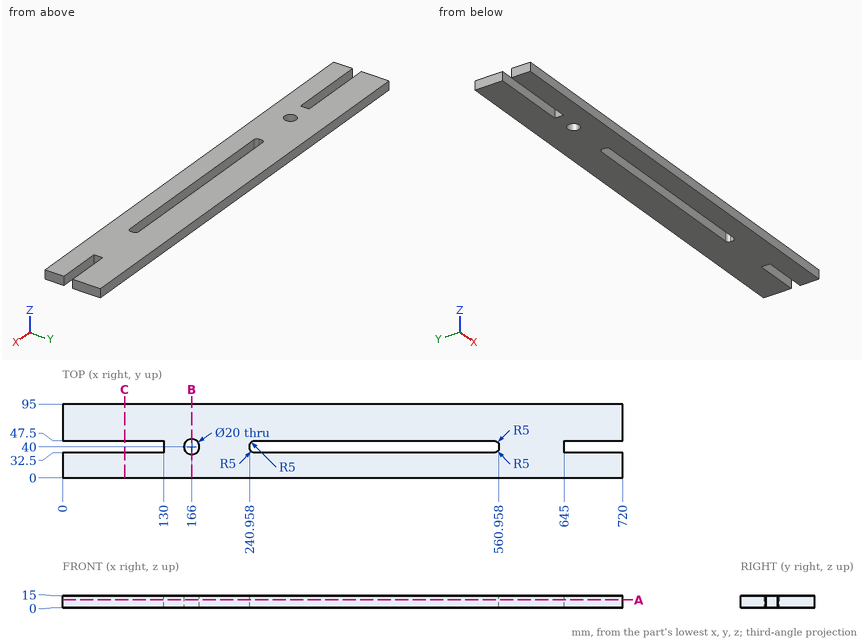
Design review of the part shown in the three views and the two pictorial views. Dimensions are in mm from the part's minimum x, y and z. Coordinates: 2 decimals unless noted, no trailing zeros. Loops run counter-clockwise (first coordinate to the right, second up) from the corner with the lowest first, then second, coordinate; pieces in that order, holes last. Notation, with made-up numbers: M 14,-21 L 63,-21 A17 cw 63,9 Z; hole C 47.5,51.5 d2. An arc over 180 degrees is marked long. Put each result on its own line as item: value. Start each with the question number.
Q1. Add section B-B (x = 166). Write out the cut boundary in (y, z).
Q2. Add section A-A (z = 9.75). Write out the cut boundary in (x, y).
Q3. Clearance check with flat-ended pins moving along their axes: pin 1 (4 mm diameter, centred on y = 41, z = 9, fed in from +X); pin 2 (1.5 mm diameter, centred on y = 40.5, z = 7.5, fed in from -X). State where each tip first meets the part, or that it passes through.
Q4. Wall thickness on line 1 (Y direction, x = 166, z = 5.5); line 2 (Y direction, x = 251, z = 3.25); line 3 (X direction, y = 36, z = 14.5) (1 decimal): over which ranges is each line inside the solid? List them lowest first.
Q5. Add section C-C (x = 80). Write out the cut boundary in (y, z), and give its area (3 significant figures).
Answers:
1. outline: M 0,0 L 30,0 L 30,15 L 0,15 Z; M 50,0 L 95,0 L 95,15 L 50,15 Z
2. outline: M 0,0 L 720,0 L 720,32.5 L 645,32.5 L 645,47.5 L 720,47.5 L 720,95 L 0,95 L 0,47.5 L 130,47.5 L 130,32.5 L 0,32.5 Z; hole C 166,40 d20; hole M 240.96,37.5 A5 ccw 245.96,32.5 L 555.96,32.5 A5 ccw 560.96,37.5 L 560.96,42.5 A5 ccw 555.96,47.5 L 245.96,47.5 A5 ccw 240.96,42.5 Z
3. pin 1: stops at x = 645
3. pin 2: stops at x = 130
4. line 1: y = 0 to 30, 50 to 95
4. line 2: y = 0 to 32.5, 47.5 to 95
4. line 3: x = 130 to 156.8, 175.2 to 241.2, 560.7 to 645
5. outline: M 0,0 L 32.5,0 L 32.5,15 L 0,15 Z; M 47.5,0 L 95,0 L 95,15 L 47.5,15 Z
5. area: 1,200 mm^2
